from build123d import *

# Parameters (mm, degrees)
SKETCH1_R           = 10.05
BOSS_EXTRUDE1_DEPTH = 1.746
SKETCH2_R           = 12.55
BOSS_EXTRUDE2_DEPTH = 4
SKETCH3_R           = 4.5
CUT_EXTRUDE1_DEPTH  = 6.746
SKETCH4_R           = 2.55
CUT_EXTRUDE2_DEPTH  = 2.5
SKETCH5_R           = 2
CUT_EXTRUDE3_DEPTH  = 0.3
CHAMFER1_SIZE       = 0.3
SKETCH6_R           = 1.1
CUT_EXTRUDE4_DEPTH  = 2.5
CUT_EXTRUDE5_DEPTH  = 1.7
CUT_EXTRUDE6_DEPTH  = 3
CIRPATTERN1_COUNT   = 3
FILLET1_R           = 0.5
SKETCH12_R          = 12.55
BOSS_EXTRUDE3_DEPTH = 1.5
SKETCH13_R          = 1.7
CUT_EXTRUDE7_DEPTH  = 3.5
CUT_EXTRUDE9_DEPTH  = 1.9
CHAMFER2_SIZE       = 0.3
SKETCH16_R          = 5.25
CUT_EXTRUDE10_DEPTH = 0.5
SKETCH18_R          = 1.2
BOSS_EXTRUDE4_DEPTH = 0.1


with BuildPart() as part:
    # Sketch1 → Boss-Extrude1 (new body)
    with BuildSketch(Plane(origin=(0, 0, 0), x_dir=(1, 0, 0), z_dir=(0, 1, 0))):
        Circle(SKETCH1_R)
    extrude(amount=BOSS_EXTRUDE1_DEPTH)

    # Sketch2 → Boss-Extrude2 (add)
    with BuildSketch(Plane(origin=(0, 1.746, 0), x_dir=(1, 0, 0), z_dir=(0, 1, 0))):
        Circle(SKETCH2_R)
    extrude(amount=BOSS_EXTRUDE2_DEPTH)

    # Sketch3 → Cut-Extrude1 (cut, through all)
    with BuildSketch(Plane.XZ):
        Circle(SKETCH3_R)
    extrude(amount=-CUT_EXTRUDE1_DEPTH, mode=Mode.SUBTRACT)

    # Sketch4 → Cut-Extrude2 (cut)
    with BuildSketch(Plane.XZ):
        with Locations((0, 6.75)):
            Circle(SKETCH4_R)
        with Locations((5.845671476, -3.375)):
            Circle(SKETCH4_R)
        with Locations((-5.845671476, -3.375)):
            Circle(SKETCH4_R)
    extrude(amount=-CUT_EXTRUDE2_DEPTH, mode=Mode.SUBTRACT)

    # Sketch5 → Cut-Extrude3 (cut)
    with BuildSketch(Plane.XZ.offset(-2.5)):
        with Locations((0, 6.75)):
            Circle(SKETCH5_R)
        with Locations((-5.845671476, -3.375)):
            Circle(SKETCH5_R)
        with Locations((5.845671476, -3.375)):
            Circle(SKETCH5_R)
    extrude(amount=-CUT_EXTRUDE3_DEPTH, mode=Mode.SUBTRACT)

    # Chamfer1
    chamfer1_edges = [part.edges().sort_by_distance(p)[0] for p in [
        (0, 0, 9.3),
        (8.054036255, 0, -4.65),
        (-8.054036255, 0, -4.65),
    ]]
    chamfer(chamfer1_edges, length=CHAMFER1_SIZE)

    # Sketch6 → Cut-Extrude4 (cut)
    with BuildSketch(Plane.XZ):
        with Locations((6.711696879, 3.875)):
            Circle(SKETCH6_R)
        with Locations((0, -7.75)):
            Circle(SKETCH6_R)
        with Locations((-6.711696879, 3.875)):
            Circle(SKETCH6_R)
    extrude(amount=-CUT_EXTRUDE4_DEPTH, mode=Mode.SUBTRACT)

    # Sketch10 → Revolve1 (revolve)
    with BuildSketch(Plane.XY):
        Polygon((10.05, 0), (10.05, 1.746), (12.55, 1.746), (13.062080355, 1.450350269), (10.55, 0), align=None)
    revolve(axis=Axis((0, 5.746, 0), (0, -1, 0)))

    # Sketch7 → Cut-Extrude5 (cut)
    with BuildSketch(Plane(origin=(0, 1.3, 0), x_dir=(-1, 0, 0), z_dir=(0, -1, 0))):
        Polygon((-1.975, 8.890266782), (-1.975, 18.890266782), (1.975, 18.890266782), (1.975, 8.890266782), (1.975, 6.609733218), (0, 5.469466437), (-1.975, 6.609733218), align=None)
    cut_extrude5 = extrude(amount=-CUT_EXTRUDE5_DEPTH, mode=Mode.SUBTRACT)

    # Sketch11 → Cut-Extrude6 (cut)
    with BuildSketch(Plane.XZ):
        with BuildLine():
            Line((-1.975, -19.854028364), (-1.975, -9.854028364))
            ThreePointArc((-1.975, -9.854028364), (0, -10.05), (1.975, -9.854028364))
            Line((1.975, -9.854028364), (1.975, -19.854028364))
            ThreePointArc((1.975, -19.854028364), (0, -19.952019128), (-1.975, -19.854028364))
        make_face()
    cut_extrude6 = extrude(amount=-CUT_EXTRUDE6_DEPTH, mode=Mode.SUBTRACT)

    # CirPattern1: Cut-Extrude5, Cut-Extrude6 ×3 about axis
    cirpattern1_axis = Axis((0, 0, 0), (0, 1, 0))
    for i in range(1, CIRPATTERN1_COUNT):
        add(cut_extrude5.rotate(cirpattern1_axis, i * 360 / CIRPATTERN1_COUNT), mode=Mode.SUBTRACT)
        add(cut_extrude6.rotate(cirpattern1_axis, i * 360 / CIRPATTERN1_COUNT), mode=Mode.SUBTRACT)

    # Fillet1
    fillet1_edges = [part.edges().sort_by_distance(p)[0] for p in [
        (0, 1.746, 12.55),
        (9.546956321, 1.746, -8.146049656),
        (-10.868618817, 1.746, -6.275),
    ]]
    fillet(fillet1_edges, radius=FILLET1_R)

    # Sketch12 → Boss-Extrude3 (add)
    with BuildSketch(Plane(origin=(0, 5.746, 0), x_dir=(1, 0, 0), z_dir=(0, 1, 0))):
        Circle(SKETCH12_R)
    extrude(amount=BOSS_EXTRUDE3_DEPTH)

    # Sketch13 → Cut-Extrude7 (cut)
    with BuildSketch(Plane(origin=(0, 7.246, 0), x_dir=(1, 0, 0), z_dir=(0, 1, 0))):
        with Locations((0, -8)):
            Circle(SKETCH13_R)
        with Locations((-8, 0)):
            Circle(SKETCH13_R)
        with Locations((0, 8)):
            Circle(SKETCH13_R)
        with Locations((8, 0)):
            Circle(SKETCH13_R)
    extrude(amount=-CUT_EXTRUDE7_DEPTH, mode=Mode.SUBTRACT)

    # Sketch15 → Cut-Extrude9 (cut)
    with BuildSketch(Plane(origin=(0, 3.746, 0), x_dir=(1, 0, 0), z_dir=(0, 1, 0))):
        Polygon((-2.75, -10.75), (-2.75, -15.75), (2.75, -15.75), (2.75, -10.75), (2.75, -5.25), (-2.75, -5.25), align=None)
        Polygon((-15.75, -2.75), (-10.75, -2.75), (-5.25, -2.75), (-5.25, 2.75), (-10.75, 2.75), (-15.75, 2.75), align=None)
        Polygon((-2.75, 15.75), (-2.75, 10.75), (-2.75, 5.25), (2.75, 5.25), (2.75, 10.75), (2.75, 15.75), align=None)
        Polygon((15.75, 2.75), (10.75, 2.75), (5.25, 2.75), (5.25, -2.75), (10.75, -2.75), (15.75, -2.75), align=None)
    extrude(amount=CUT_EXTRUDE9_DEPTH, mode=Mode.SUBTRACT)

    # Chamfer2
    chamfer2_edges = [part.edges().sort_by_distance(p)[0] for p in [
        (-12.55, 7.246, 0),
    ]]
    chamfer(chamfer2_edges, length=CHAMFER2_SIZE)

    # Sketch16 → Cut-Extrude10 (cut)
    with BuildSketch(Plane.XZ):
        with Locations((0, 6.75)):
            Circle(SKETCH16_R)
        with Locations((-5.845671476, -3.375)):
            Circle(SKETCH16_R)
        with Locations((5.845671476, -3.375)):
            Circle(SKETCH16_R)
    extrude(amount=-CUT_EXTRUDE10_DEPTH, mode=Mode.SUBTRACT)

    # Sketch18 → Boss-Extrude4 (add)
    with BuildSketch(Plane(origin=(0, 1.3, 0), x_dir=(1, 0, 0), z_dir=(0, 1, 0))):
        with Locations((6.711696879, -3.875)):
            Circle(SKETCH18_R)
        with Locations((0, 7.75)):
            Circle(SKETCH18_R)
        with Locations((-6.711696879, -3.875)):
            Circle(SKETCH18_R)
    extrude(amount=-BOSS_EXTRUDE4_DEPTH)


solid = part.part
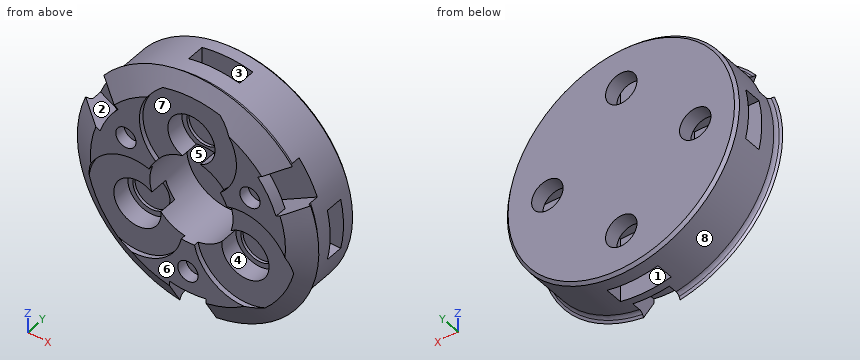
Work out the finished part from the listing and answer in its coordinate system (mm). Face numbers are marked on the shaded views. A direction names the side the tool comes from. Round coordinates to 2 decimals unless told otherwise and drop trailing zeros. Order: outer loops, then holes, each group sorted by start corner. A loop starts at its lowest first (then second) coordinate and runs counter-clockwise, first axis right, second up. Notation, with made-up numbers: M 49.5,-6.5 L 90.5,-6.5 A25 ccw 90.5,14.5 Z; hole C 16.5,-4.5 d1. An arc over 180 degrees is marked long. Put each result on its own line as item: value. Start each with the question number.
Q1. Straight lines are drawn through the part: L1, parallel to Z at x = 0, y = 6.1; L2, parallel to Y at x = 5.5, z = -1; L3, parallel to Y at x = 7, z = 6. For each, find the intervals that lie inside material, in ascending order. Write a range as [from, to].
Q2. For a pull along Z with two mould halves and no side action, classify the marked faces 5, 6, 7 and 8 as pulls with the +Z half, pulls with the -Z half, needs draft (parallel to the pull), parting line crosses it, or undercut.
Q3. Section A-A, the plane y = 5.25 is taken. Write down the section's boundary in (x, z) (3 decimals).
Q4. A tool of negligible diameter and unlimited length cuts with its end or side. For the marked faces 1, 2, 3 and 4, from which of +Z, -Z, +X, -X, +Y, -Y can it reach the whole face along a straight path? Write none if from no direction.
Q5. Flat-ended cylindrical pins translate along their axes: pin 1 (0.7 mm diameter, centred on x = -6.5, z = 4, fed in from -Y); pin 2 (5 mm diameter, centred on x = -2.5, z = 7.5, fed in from -Y); pin 3 (0.6 mm diameter, centred on x = -8.5, y = 5, fed in from +Z). Find the tip coordinate at first contact, or state that the pin passes through.
Findings below:
1. L1: z = [-12.55, -9.7], [-6.3, 6.3], [9.7, 12.55]
1. L2: y = [2.5, 3.75], [5.65, 7.25]
1. L3: y = [0, 1.3], [3, 7.25]
2. face 5: undercut
2. face 6: needs draft
2. face 7: undercut
2. face 8: parting line crosses it
3. outline: M -12.245,-2.75 A12.55 ccw -2.75,-12.245 L -2.75,-5.25 L 2.75,-5.25 L 2.75,-12.245 A12.55 ccw 12.245,-2.75 L 5.25,-2.75 L 5.25,2.75 L 12.245,2.75 A12.55 ccw 2.75,12.245 L 2.75,5.25 L -2.75,5.25 L -2.75,12.245 A12.55 ccw -12.245,2.75 L -5.25,2.75 L -5.25,-2.75 Z; hole C 0,0 d9
4. face 1: -Z
4. face 2: none
4. face 3: +Z
4. face 4: -Y
5. pin 1: stops at y = 1.2
5. pin 2: stops at y = 0.5
5. pin 3: stops at z = 9.5
